The model under review builds one solid part; all positions refer to its coordinate system, in mm. A direction names the side the tool comes from. Round coordinates to 2 decimals unless told otherwise and drop trailing zeros. Write each loop counter-clockwise with the first axis right and the second up, starting at its lowest first coordinate (ties: lowest second). Pieces come first, ordered by that corner, then holes. Notation, with made-up numbers: (-33.5, -40) - (-25.5, -40) arc R21 ccw to (-25.5, -26) - close; hole circle Ø9 at (-12, -3.5). An arc over 180 degrees is marked (long way). Write each question's results on one line, items separated by ' | '.
```python
from build123d import *

# Parameters (mm, degrees)
F0_W     = 275
F0_H     = 275
F0_W_2   = 50.5
F0_H_2   = 50.5
F1_DEPTH = 50
F2_DEPTH = 400
F3_SIZE  = 2
F4_R     = 2
F5_R     = 1


with BuildPart() as f1:
    # F0 (on Top) → F1 (new body)
    with BuildSketch(Plane.XY):
        with Locations((-137.5, -137.5)):
            Rectangle(F0_W, F0_H)
        with Locations((-247.65, -247.65)):
            Rectangle(F0_W_2, F0_H_2, mode=Mode.SUBTRACT)
        with Locations((-247.65, -247.65)):
            Rectangle(F0_W_2, F0_H_2)
    extrude(amount=F1_DEPTH)

    # F0 (on Top) → F2 (join)
    with BuildSketch(Plane.XY):
        with Locations((-247.65, -247.65)):
            Rectangle(F0_W_2, F0_H_2)
    extrude(amount=-F2_DEPTH)

    # F3
    f3_edges = [f1.edges().sort_by_distance(p)[0] for p in [
        (-272.9, -247.65, -400),
        (-247.65, -272.9, -400),
        (-222.4, -247.65, -400),
        (-247.65, -222.4, -400),
    ]]
    chamfer(f3_edges, length=F3_SIZE)

    # F4
    f4_edges = [f1.edges().sort_by_distance(p)[0] for p in [
        (-272.9, -272.9, -199),
        (-222.4, -272.9, -199),
        (-272.9, -222.4, -199),
        (-222.4, -222.4, -199),
    ]]
    fillet(f4_edges, radius=F4_R)

    # F5
    f5_edges = [f1.edges().sort_by_distance(p)[0] for p in [
        (-275, -137.5, 50),
        (-275, -137.5, 0),
        (-275, -275, 25),
        (-137.5, -275, 50),
        (-137.5, -275, 0),
    ]]
    fillet(f5_edges, radius=F5_R)

    # F6: F1 across face


with BuildPart() as f1_1:
    add(f1.part)
    add(f1.part.mirror(Plane(origin=(0, -137.4957148019, 25), x_dir=(0, 1, 0), z_dir=(1, 0, 0))))

    # F7: F1 across face


with BuildPart() as f1_2:
    add(f1_1.part)
    add(f1_1.part.mirror(Plane(origin=(0, 0, 25), x_dir=(-1, 0, 0), z_dir=(0, 1, 0))))


solid = f1_2.part
```
Q1. Insertion check: P1, Ø14, axis at y = 258, z = -134, coming from the +X side; P2, Ø23, axis at x = -258.5, z = -103.5, coming from the +Y side; P3, Ø6, axis at x = -205.5, y = -44.5, coming from the -Z side. Each pin has a flat end and moves straight along its axis. Give the tip position at first contact, or say it passes through.
Evaluation:
P1: stops at x = 272.9 | P2: stops at y = 272.9 | P3: stops at z = 0
Q2. The part is to be moulded in two halves that separate along X. For faces 1 (the flat face through (-275, 4, 25)), 2 (the flat face through (-222.4, 248, -196)), 3 (the flat face through (-248, -247, -400)), say which applies: released by +X, released by -X, zero draft, split by the parting line, or undercut.
Evaluation:
face 1: released by -X | face 2: undercut | face 3: zero draft
Q3. We need section A-A (y = -145). State the section outline as (x, z) points.
Evaluation:
outline: (-275, 1) arc R1 ccw to (-274, 0) - (274, 0) arc R1 ccw to (275, 1) - (275, 49) arc R1 ccw to (274, 50) - (-274, 50) arc R1 ccw to (-275, 49) - close
Q4. We need section C-C (x = -235). State the section outline as (y, z) points, plus the area to 3 significant figures.
Evaluation:
outline: (-275, 1) arc R1 ccw to (-274, 0) - (-272.9, 0) - (-272.9, -398) - (-270.9, -400) - (-224.4, -400) - (-222.4, -398) - (-222.4, 0) - (222.4, 0) - (222.4, -398) - (224.4, -400) - (270.9, -400) - (272.9, -398) - (272.9, 0) - (274, 0) arc R1 ccw to (275, 1) - (275, 49) arc R1 ccw to (274, 50) - (-274, 50) arc R1 ccw to (-275, 49) - close | area: 67,900 mm^2
Q5. Tool access review of faces 4 (the flat face through (272.9, 248, -196)), 5 (the flat face through (-248, 272.9, -196)), 6 (the flat face through (248, -222.4, -196)): name each direction out of +Z, -Z, +X, -X, +Y, -Y from which nothing blocks a thin tool from reaching the whole face with its end or side.
Evaluation:
face 4: -Z, +X, +Y, -Y | face 5: -Z, +X, -X, +Y | face 6: -Z, +X, -X
Q6. For probe 1 along X at (y, z) = (-246.5, -352.5); probe 2 along Z at (x, y) = (-187.5, 85), list the stretches that pass through material, from the lowest coordinate up.
Evaluation:
probe 1: x = -272.9 to -222.4, 222.4 to 272.9 | probe 2: z = 0 to 50
Q7. We need section B-B (z = -196). State how many separate pieces and enclosed holes the cut face has, plus the area to 3 significant figures.
Evaluation:
separate pieces: 4 | enclosed holes: 0 | area: 10,200 mm^2
